```python
from build123d import *

# Parameters (mm, degrees)
EXTRUDE_1_DEPTH     = 20
SKETCH_2_W          = 20
SKETCH_2_H          = 10
CUT_EXTRUDE_1_DEPTH = 1.5
SKETCH_3_R          = 1.55
CUT_EXTRUDE_2_DEPTH = 15
SKETCH_4_R          = 1.55
CUT_EXTRUDE_5_DEPTH = 5
SKETCH_6_R          = 1.55
CUT_EXTRUDE_6_DEPTH = 10


with BuildPart() as part:
    # 草图1 → 凸台-拉伸1 (new body)
    with BuildSketch(Plane.XY):
        with BuildLine():
            Line((-9, 0), (-9, 30))
            Line((-9, 30), (9, 30))
            Line((9, 30), (9, 0))
            ThreePointArc((9, 0), (0, 9), (-9, 0))
        make_face()
    extrude(amount=EXTRUDE_1_DEPTH)

    # 草图2 → 切除-拉伸1 (cut)
    with BuildSketch(Plane.ZY.offset(9)):
        with Locations((10, 20)):
            Rectangle(SKETCH_2_W, SKETCH_2_H)
    cut_extrude_1 = extrude(amount=-CUT_EXTRUDE_1_DEPTH, mode=Mode.SUBTRACT)

    # 镜向1: 切除-拉伸1 across plane
    add(cut_extrude_1.mirror(Plane(origin=(0, 0, 0), x_dir=(0, 0, 1), z_dir=(1, 0, 0))), mode=Mode.SUBTRACT)

    # 草图3 → 切除-拉伸2 (cut)
    with BuildSketch(Plane(origin=(7.5, 0, 0), x_dir=(0, 0, -1), z_dir=(1, 0, 0))):
        with Locations((-6, 22)):
            Circle(SKETCH_3_R)
        with Locations((-10, 18)):
            Circle(SKETCH_3_R)
    extrude(amount=-CUT_EXTRUDE_2_DEPTH, mode=Mode.SUBTRACT)

    # 草图4 → 切除-拉伸5 (cut)
    with BuildSketch(Plane(origin=(0, 30, 0), x_dir=(1, 0, 0), z_dir=(0, 1, 0))):
        with Locations((-5, -5)):
            Circle(SKETCH_4_R)
        with Locations((5, -5)):
            Circle(SKETCH_4_R)
        with Locations((5, -15)):
            Circle(SKETCH_4_R)
        with Locations((-5, -15)):
            Circle(SKETCH_4_R)
    extrude(amount=-CUT_EXTRUDE_5_DEPTH, mode=Mode.SUBTRACT)

    # 草图6 → 切除-拉伸6 (cut)
    with BuildSketch(Plane(origin=(0, 30, 0), x_dir=(1, 0, 0), z_dir=(0, 1, 0))):
        with Locations((-5, -15)):
            Circle(SKETCH_6_R)
        with Locations((5, -15)):
            Circle(SKETCH_6_R)
    extrude(amount=-CUT_EXTRUDE_6_DEPTH, mode=Mode.SUBTRACT)


solid = part.part
```
Here's how the part is built. I have some questions about the finished solid (model axes, mm). A direction names the side the tool comes from. Give positions to 0.01 mm unless a question says otherwise; leave off trailing zeros. Write each loop counter-clockwise with the first axis right and the second up, starting at its lowest first coordinate (ties: lowest second). Pieces come first, ordered by that corner, then holes. Notation, with made-up numbers: M 35,38.25 L 74,38.25 A14 ccw 74,50.25 Z; hole C 25.5,44 d1. An arc over 180 degrees is marked long. Put each result on its own line as item: value. Start each with the question number.
Item 1: On a 3-axis mill with a long thin cutter (end or side, diameter ignored), from which of +Z, -Z, +X, -X, +Y, -Y can I reach the whole of each face in a straight line? I mean faces 4 (the flat face through (8, 15, 10)), 5 (the flat face through (-8, 15, 10)), 6 (the flat face through (5, 25, 5)). Say none if no direction works.
Item 2: Will these pins go through, and if not, where does the flat tip stop? pin 1 (3.5 mm diameter, centred on x = 5, z = 15, fed in from -Y); pin 2 (4 mm diameter, centred on x = -5, z = 5, fed in from -Y); pin 3 (3 mm diameter, centred on x = -5, z = 15, fed in from +Y); pin 4 (2.5 mm diameter, centred on y = 22, z = 6, fed in from -X).
Item 3: If we section it at A-A, the plane y = 22: Write out the boundary of the cut face in (x, z).
Item 4: I need wall thicknesses on L1, parallel to X at y = 25.75, z = 15; L2, parallel to Z at x = -5, y = 27.75; L3, parallel to Z at x = -4.25, y = 26.25. Which ranges of each line are inside material? Lowest first, please. Write a range as from..to.
Item 5: Thinking about a two-plate mould opening in Z: for faces 1 (the flat face through (0, 19, 0)), 2 (the flat face through (-9, 7, 10)), 3 (the flat face through (5, 20, 15)), which applies, +Z half, -Z half, draft (parallel to the pull), parting line (faces both ways), or undercut?
Item 6: If we section it at C-C, the plane z = 15: Write out the boundary of the cut face in (x, y).
Item 7: If we section it at D-D, the plane z = 6: Write out the boundary of the cut face in (x, y).
Item 8: If we section it at B-B, the plane y = 25.75: Write out the boundary of the cut face in (x, z), then the cut area to 3 significant figures.
Values:
1. face 4: +Z, -Z, +X
1. face 5: +Z, -Z, -X
1. face 6: +Y
2. pin 1: y = 5.95
2. pin 2: y = 5.66
2. pin 3: y = 20
2. pin 4: through
3. outline: M -7.5,0 L 7.5,0 L 7.5,4.45 L -7.5,4.45 Z; M -7.5,7.55 L 7.5,7.55 L 7.5,20 L -7.5,20 Z; hole C -5,15 d3.1; hole C 5,15 d3.1
4. L1: -9..-6.55, -3.45..3.45, 6.55..9
4. L2: 0..3.45, 6.55..13.45, 16.55..20
4. L3: 0..3.64, 6.36..13.64, 16.36..20
5. face 1: -Z half
5. face 2: draft
5. face 3: undercut
6. outline: M -9,0 A9 cw 9,0 L 9,15 L 7.5,15 L 7.5,25 L 9,25 L 9,30 L 6.55,30 L 6.55,20 L 3.45,20 L 3.45,30 L -3.45,30 L -3.45,20 L -6.55,20 L -6.55,30 L -9,30 L -9,25 L -7.5,25 L -7.5,15 L -9,15 Z
7. outline: M -9,0 A9 cw 9,0 L 9,15 L 7.5,15 L 7.5,20.45 L -7.5,20.45 L -7.5,15 L -9,15 Z; M -9,25 L -7.5,25 L -7.5,23.55 L 7.5,23.55 L 7.5,25 L 9,25 L 9,30 L 6.18,30 L 6.18,25 L 3.82,25 L 3.82,30 L -3.82,30 L -3.82,25 L -6.18,25 L -6.18,30 L -9,30 Z
8. outline: M -9,0 L 9,0 L 9,20 L -9,20 Z; hole C -5,5 d3.1; hole C -5,15 d3.1; hole C 5,5 d3.1; hole C 5,15 d3.1
8. area: 330 mm²
